```python
from build123d import *

# Parameters (mm, degrees)
SKETCH1_W           = 40
SKETCH1_H           = 35
SKETCH1_R           = 12
SKETCH1_R_2         = 1.5
SKETCH1_R_3         = 4.1
BOSS_EXTRUDE1_DEPTH = 3
FILLET1_R           = 3


with BuildPart() as part:
    # Sketch1 → Boss-Extrude1 (new body)
    # profile 1 of 2: a face of its own
    with BuildSketch(Plane(origin=(0, 0, 0), x_dir=(1, 0, 0), z_dir=(0, 1, 0))):
        with Locations((15, 12.5)):
            Rectangle(SKETCH1_W, SKETCH1_H)
        with Locations((15, 12.5)):
            Circle(SKETCH1_R, mode=Mode.SUBTRACT)
        with Locations(Location((0, 25, 0), (0, 0, 270))):
            Circle(SKETCH1_R_2, mode=Mode.SUBTRACT)
        with Locations(Location((30, 25, 0), (0, 0, 270))):
            Circle(SKETCH1_R_2, mode=Mode.SUBTRACT)
        with Locations(Location((30, 0, 0), (0, 0, 270))):
            Circle(SKETCH1_R_2, mode=Mode.SUBTRACT)
        with Locations(Location((0, 0, 0), (0, 0, 270))):
            Circle(SKETCH1_R_2, mode=Mode.SUBTRACT)
    # profile 2 of 2: a face of its own
    with BuildSketch(Plane(origin=(0, 0, 0), x_dir=(1, 0, 0), z_dir=(0, 1, 0))):
        with Locations((15, 12.5)):
            Circle(SKETCH1_R)
        with Locations(Location((15, 12.5, 0), (0, 0, 270))):
            Circle(SKETCH1_R_3, mode=Mode.SUBTRACT)
    extrude(amount=BOSS_EXTRUDE1_DEPTH)

    # Fillet1
    fillet1_edges = [part.edges().sort_by_distance(p)[0] for p in [
        (35, 1.5, -30),
        (35, 1.5, 5),
        (-5, 1.5, 5),
        (-5, 1.5, -30),
    ]]
    fillet(fillet1_edges, radius=FILLET1_R)


solid = part.part
```
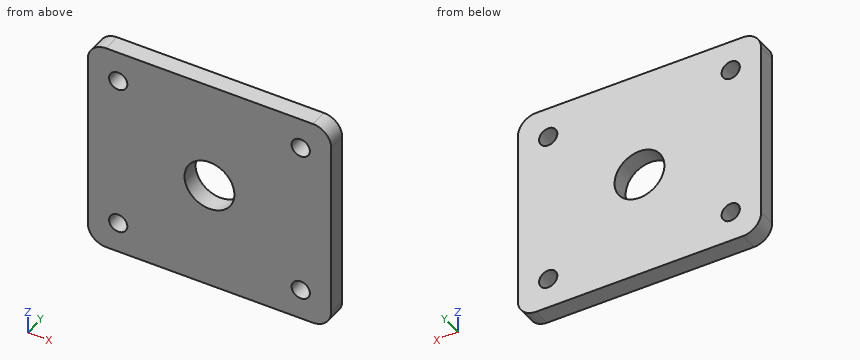
Can you work these out from the model? Positions are in its coordinate system, mm. Coordinates: 2 decimals unless noted, no trailing zeros. Loops run counter-clockwise (first coordinate to the right, second up) from the corner with the lowest first, then second, coordinate; pieces in that order, holes last. Notation, with made-up numbers: (-36.75, 72) -> (-8.75, 72) arc R19 ccw to (-8.75, 80) -> close; hole circle Ø7 at (0, 30.25). An arc over 180 degrees is marked (long way). Answer as a JSON object with one key per item and string values.
1) If I drill on line 1 (X direction, y = 2.4, z = 0); line 2 (X direction, y = 2, z = -12.5); line 3 (X direction, y = 0.95, z = 1), over which ranges is the centre line in solid material (lowest first)?
Results:
{"line 1": "x = -5 to -1.5, 1.5 to 28.5, 31.5 to 35", "line 2": "x = -5 to 10.9, 19.1 to 35", "line 3": "x = -5 to -1.12, 1.12 to 28.88, 31.12 to 35"}
2) Imagine slicing it at B-B (x = 30). Please give me the cut outline in (y, z).
Results:
{"outline": "(0, -30) -> (3, -30) -> (3, -26.5) -> (0, -26.5) -> close; (0, -23.5) -> (3, -23.5) -> (3, -1.5) -> (0, -1.5) -> close; (0, 1.5) -> (3, 1.5) -> (3, 5) -> (0, 5) -> close"}
3) Imagine slicing it at C-C (z = 0). Please give me the cut outline in (x, y), then the cut area to 3 significant figures.
Results:
{"outline": "(-5, 0) -> (-1.5, 0) -> (-1.5, 3) -> (-5, 3) -> close; (1.5, 0) -> (28.5, 0) -> (28.5, 3) -> (1.5, 3) -> close; (31.5, 0) -> (35, 0) -> (35, 3) -> (31.5, 3) -> close", "area": "102 mm^2"}
4) For P1, Ø5, axis at x = 0, z = 0, coming from the +Y side, with a flat end and sliding along its axis, tell me the tip position at first contact or that it passes through.
Results:
{"P1": "stops at y = 3"}
5) Imagine slicing it at D-D (y = 1.8). Please give me the cut outline in (x, z), then the cut area to 3 significant figures.
Results:
{"outline": "(-5, -27) arc R3 ccw to (-2, -30) -> (32, -30) arc R3 ccw to (35, -27) -> (35, 2) arc R3 ccw to (32, 5) -> (-2, 5) arc R3 ccw to (-5, 2) -> close; hole circle Ø3 at (0, -25); hole circle Ø3 at (0, 0); hole circle Ø8.2 at (15, -12.5); hole circle Ø3 at (30, -25); hole circle Ø3 at (30, 0)", "area": "1,310 mm^2"}
6) Imagine slicing it at A-A (z = -12.5). Please give me the cut outline in (x, y).
Results:
{"outline": "(-5, 0) -> (10.9, 0) -> (10.9, 3) -> (-5, 3) -> close; (19.1, 0) -> (35, 0) -> (35, 3) -> (19.1, 3) -> close"}
